from build123d import *

# Parameters (mm, degrees)
F0_W     = 145
F0_H     = 60
F1_DEPTH = 15
F4_DEPTH = 12
F3_R     = 26
F5_DEPTH = 16
F3_R_2   = 16
F6_DEPTH = 21
F7_DEPTH = 4
F8_DEPTH = 4


with BuildPart() as f1:
    # F0 (on Top) → F1 (new body)
    with BuildSketch(Plane.XY):
        Rectangle(F0_W, F0_H)
        with BuildLine():
            ThreePointArc((37.5, 1), (44.5, -6), (37.5, -13))
            Line((37.5, -13), (-37.5, -13))
            ThreePointArc((-37.5, -13), (-44.5, -6), (-37.5, 1))
            Line((-37.5, 1), (37.5, 1))
        make_face(mode=Mode.SUBTRACT)
    extrude(amount=F1_DEPTH)

    # F3 (on offset) → F4 (join)
    with BuildSketch(Plane(origin=(0, 30, 0), x_dir=(-1, 0, 0), z_dir=(0, 1, 0))):
        with BuildLine():
            Line((12.092110391, 119.3122868922), (-72.5, 15))
            Line((-72.5, 15), (72.5, 15))
            Line((72.5, 15), (72.5, 97.8967932859))
            ThreePointArc((72.5, 97.8967932859), (27.1392836208, 65.8509804026), (12.092110391, 119.3122868922))
        make_face()
    extrude(amount=-F4_DEPTH)

    # F3 (on offset) → F5 (join)
    with BuildSketch(Plane(origin=(0, 30, 0), x_dir=(-1, 0, 0), z_dir=(0, 1, 0))):
        with BuildLine():
            ThreePointArc((72.5, 97.8967932859), (49.8607163792, 129.9426061692), (12.092110391, 119.3122868922))
            ThreePointArc((12.092110391, 119.3122868922), (27.1392836208, 65.8509804026), (72.5, 97.8967932859))
        make_face()
        with Locations((38.5, 97.8967932859)):
            Circle(F3_R, mode=Mode.SUBTRACT)
    extrude(amount=-F5_DEPTH)

    # F3 (on offset) → F6 (join)
    with BuildSketch(Plane(origin=(0, 30, 0), x_dir=(-1, 0, 0), z_dir=(0, 1, 0))):
        with Locations((38.5, 97.8967932859)):
            Circle(F3_R)
        with Locations((38.5, 97.8967932859)):
            Circle(F3_R_2, mode=Mode.SUBTRACT)
    extrude(amount=-F6_DEPTH)

    # F3 (on offset) → F7 (join)
    with BuildSketch(Plane(origin=(0, 30, 0), x_dir=(-1, 0, 0), z_dir=(0, 1, 0))):
        with BuildLine():
            ThreePointArc((72.5, 97.8967932859), (49.8607163792, 129.9426061692), (12.092110391, 119.3122868922))
            ThreePointArc((12.092110391, 119.3122868922), (27.1392836208, 65.8509804026), (72.5, 97.8967932859))
        make_face()
        with Locations((38.5, 97.8967932859)):
            Circle(F3_R, mode=Mode.SUBTRACT)
    extrude(amount=F7_DEPTH)

    # F3 (on offset) → F8 (join)
    with BuildSketch(Plane(origin=(0, 30, 0), x_dir=(-1, 0, 0), z_dir=(0, 1, 0))):
        with Locations((38.5, 97.8967932859)):
            Circle(F3_R)
        with Locations((38.5, 97.8967932859)):
            Circle(F3_R_2, mode=Mode.SUBTRACT)
    extrude(amount=F8_DEPTH)


solid = f1.part
Could you check a few things on this model? Use its own coordinates, in mm. A direction names the side the tool comes from. Coordinates: 2 decimals unless noted, no trailing zeros. Write each loop counter-clockwise with the first axis right and the second up, starting at its lowest first coordinate (ties: lowest second). Pieces come first, ordered by that corner, then holes. Notation, with made-up numbers: (-38.75, -10) - (12.25, -10) arc R34 cw to (12.25, 23) - close; hole circle Ø2 at (-2, 23). An arc over 180 degrees is marked (long way). Put each result on its own line as item: value. Start each with the question number.
Q1. I want a section at D-D on z = 101.5. Write out the boundary of the cut face in (x, y).
Q2. Which directions (+Z, -Z, +X, -X, +Y, -Y) give clear straight access to the entire face, cutting with the end or side of a thin tool? Please do faces 1 (the flat face through (-30.8, 14, 72.9)), 2 (the flat face through (-50, 9, 110)), 3 (the flat face through (1, -13, 7)), 4 (the flat face through (-1, -30, 7)).
Q3. Please list where these lines run through material, in increasing order: L1, parallel to Z at x = -38.5, y = 24.5; L2, parallel to X at y = -5.5, z = 14.5; L3, parallel to Z at x = -38.5, y = 15.75.
Q4. I want a section at A-A on x = -17.5. Write out the boundary of the cut face in (y, z).
Q5. Thinking about a two-plate mould opening in X: for faces 5 (the flat face through (-1, 7, 0)), 6 (the flat face through (-72.5, 22, 31)), 7 (the cylindrical face through (-44.5, -6.15, 7.4)), which applies, pulls with the +X half, pulls with the -X half, needs draft (parallel to the pull), parting line crosses it, or undercut?
Q6. I'm going to push flat-ended pins straight in: P1, Ø12, axis at x = 7.5, z = 7.5, coming from the +Y side; P2, Ø4, axis at x = -22.5, y = -22, coming from the -Z side; P3, Ø4, axis at x = 17, z = 24, coming from the -Y side; P4, Ø6, axis at x = -29.5, y = -22, coming from the +Z side. Where does each tip first touch, or does it pass through?
Q7. I want a section at C-C on y = 21. Write out the boundary of the cut face in (x, z), plus the area to 3 significant figures.
Q8. I want a section at B-B on z = 12. Write out the boundary of the cut face in (x, y).
Checks:
1. outline: (-72.31, 14) - (-64.25, 14) - (-64.25, 9) - (-54.09, 9) - (-54.09, 34) - (-72.31, 34) - close; (-22.91, 9) - (-12.75, 9) - (-12.75, 14) - (-4.69, 14) - (-4.69, 18) - (2.35, 18) - (2.35, 30) - (-4.69, 30) - (-4.69, 34) - (-22.91, 34) - close
2. face 1: -Y
2. face 2: +Z, +X, -X, -Y
2. face 3: +Z, -Z
2. face 4: +Z, -Z, +X, -X, -Y
3. L1: 0 to 81.9, 113.9 to 131.9
3. L2: -72.5 to -44.48, 44.48 to 72.5
3. L3: 0 to 15, 63.9 to 81.9, 113.9 to 131.9
4. outline: (-30, 0) - (-13, 0) - (-13, 15) - (-30, 15) - close; (1, 0) - (30, 0) - (30, 71.16) - (34, 71.16) - (34, 124.64) - (14, 124.64) - (14, 113.23) - (9, 113.23) - (9, 82.57) - (14, 82.57) - (14, 71.16) - (18, 71.16) - (18, 15) - (1, 15) - close
5. face 5: needs draft
5. face 6: pulls with the -X half
5. face 7: undercut
6. P1: y = 30
6. P2: z = 0
6. P3: y = 18
6. P4: z = 15
7. outline: (-72.5, 0) - (72.5, 0) - (72.5, 15) - (-12.09, 119.31) arc R34 ccw to (-72.5, 97.9) - close; hole circle Ø32 at (-38.5, 97.9)
7. area: 12,500 mm²
8. outline: (-72.5, -30) - (72.5, -30) - (72.5, 30) - (-72.5, 30) - close; hole (-37.5, -13) - (37.5, -13) arc R7 ccw to (37.5, 1) - (-37.5, 1) arc R7 ccw to start
